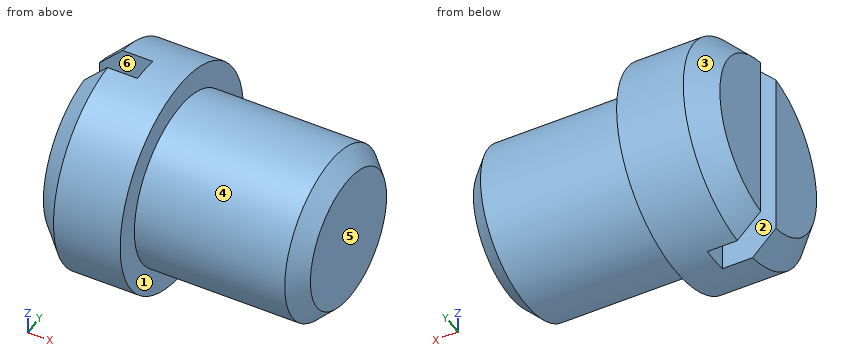
Autodesk Inventor part; units mm, degrees
ref_plane "Work Plane1" through (2.5, 0, 0) normal (0, 0, -1) x (1, 0, 0)
ref_plane "YZ Plane" through (0, 0, 0) normal (1, 0, 0) x (0, 1, 0)
ref_plane "XZ Plane" through (0, 0, 0) normal (0, 1, 0) x (-1, 0, 0)
sketch "Sketch1" plane through (0, 0, 0) normal (0, 0, 1) x (1, 0, 0)
  line L0 (-2.7, 0) -> (5, 0)
  line L1 (5, 0) -> (5, 2.5)
  line L2 (5, 2.5) -> (0, 2.5)
  line L3 (0, 2.5) -> (0, 3.25)
  line L4 (0, 3.25) -> (-2.7, 3.25)
  line L5 (-2.7, 3.25) -> (-2.7, 0)
  line L6 (-4.24, 0) -> (6.54, 0)
  line L7 (0, -0.65) -> (0, 3.9)
  dimension "d0" = 5
  dimension "d1" = 2.7
  dimension "d2" = 5
  dimension "d3" = 6.5
revolve "Body" add sketch "Sketch1" angle 360 about axis through (-2.7, 0, 0) along (1, 0, 0)
sketch "Sketch2" plane through (-2.7, 0, 0) normal (-1, 0, 0) x (0, 0, 1)
  circle A0 centre (0, 0) radius 3.25
  line L0 (-4.55, 0) -> (4.55, 0)
  line L1 (0, -4.55) -> (0, 4.55)
  line L2 (-3.25, 0.4) -> (3.25, 0.4)
  line L3 (3.25, 0.4) -> (3.25, -0.4)
  line L4 (3.25, -0.4) -> (-3.25, -0.4)
  line L5 (-3.25, -0.4) -> (-3.25, 0.4)
  line L6 (-3.25, 0) -> (3.25, 0) construction
  line L7 (0, 0.4) -> (0, -0.4) construction
  dimension "d5" = 0.8
extrude "Slot" cut sketch "Sketch2" against normal blind 1.6 contours L0 L1 L2 A0 | L3 L4 A0 | A0 L4 L1 L0 | A0 L2 L3 | L1 L4 A0 L0 | L0 A0 L2 L1 | L5 L2 A0 | A0 L4 L5
chamfer "Chamfer1" distance 0.7 angle 45 3 edges at (-2.7, -3.25, 0) (-2.7, 2.4354, -2.152) (-2.7, 2.4354, 2.152) measured on face at (-0.9, -1.3953, 2.9352)
thread "Thread"
chamfer "Chamfer2" distance 0.4908 distance2 0.4908 1 edges at (5, -2.5, 0) measured on face at (5, 0.9945, 0.5526)
ref_plane "Work Plane1" through (2.5, 0, 0) normal (0, 0, -1) x (1, 0, 0)
equation "\"d0\" = NLG"
equation "\"d1\" = KOH"
equation "\"d2\" = NND"
equation "\"d3\" = KOD"
equation "\"d5\" = SBR"
equation "\"d6\" = STI"
equation "\"d8\" = PHH"
equation "\"d16\" = PHH"
equation "\"d10\" = GEL"
equation "\"d12\" = -0.5 * GD1 + 0.5 * NND"
equation "\"d13\" = GUL"
equation "\"NND\" = 5"
equation "\"NLG\" = 5"
equation "\"GEL\" = 3.4"
equation "\"KOD\" = 6.5"
equation "\"KOH\" = 2.7"
equation "\"STI\" = 1.6"
equation "\"SBR\" = 0.8"
equation "\"GUL\" = 0.61345 * PTC"
equation "\"PHH\" = 0.7"
equation "\"GD1\" = THREADDIA - 1.2269 * PTC"
equation "\"THREADDIA\" = 5"
equation "\"TOA\" = 30deg"
equation "\"PTC\" = 0.8"
equation "\"GAL\" = 0.61345 * PTC"
properties part number "DIN 920 - M5 x 5" material "Steel, Mild"
Could you check a few things on this model? Use its own coordinates, in mm. Face numbers are marked on the shaded views. A direction names the side the tool comes from. Coordinates: 2 decimals unless noted, no trailing zeros. Order: outer loops, then holes, each group sorted by start corner. A loop starts at its lowest first (then second) coordinate and runs counter-clockwise, first axis right, second up. Notation, with made-up numbers: M 82.25,22.5 L 98.25,22.5 A16 cw 98.25,35.5 Z; hole C 45,-12.5 d6. An arc over 180 degrees is marked long. Use one line per item in the form item = value. Start each with the question number.
1. Suppose I cut it at A-A on z = 0. Write out the boundary of the cut face in (x, y), then the cut area to 3 significant figures.
2. For pin 1 (1.3 mm diameter, centred on x = -1.5, z = -0.5, fed in from +Y); pin 2 (1 mm diameter, centred on x = -1, y = 2, fed in from -Z); pin 3 (3 mm diameter, centred on x = -1, z = -2.5, fed in from -Y); pin 4 (2 mm diameter, centred on x = 1.5, y = -0.5, fed in from +Z), each with a flat end and sliding along its axis, tell me the tip position at first contact or that it passes through.
3. We'd pull the mould along Y, two halves only. Please class the marked faces 1, 2 and 3: +Y half, -Y half, draft (parallel to the pull), parting line (faces both ways), or undercut.
4. Suppose I cut it at D-D on x = 2.5. Write out the boundary of the cut face in (y, z), then the cut area to 3 significant figures.
5. On a 3-axis mill with a long thin cutter (end or side, diameter ignored), from which of +Z, -Z, +X, -X, +Y, -Y can I reach the whole of each face in a straight line? I mean the marked faces 4, 5 and 6. Say none if no direction works.
6. Please list where these lines run through material, in increasing order: line 1 (Z direction, x = 2.5, y = 0); line 2 (X direction, y = -0.25, z = -0.25); line 3 (Y direction, x = 1, z = 1.25).
7. Suppose I cut it at B-B on y = 0. Write out the boundary of the cut face in (x, z).
8. Suppose I cut it at C-C on x = -0.5. Write out the boundary of the cut face in (y, z), then the cut area to 3 significant figures.
Geometry says:
q1.outline = M -2.7,-2.55 L -2,-3.25 L 0,-3.25 L 0,-2.5 L 4.51,-2.5 L 5,-2.01 L 5,2.01 L 4.51,2.5 L 0,2.5 L 0,3.25 L -2,3.25 L -2.7,2.55 L -2.7,0.4 L -1.1,0.4 L -1.1,-0.4 L -2.7,-0.4 Z
q1.area = 40.5 mm^2
q2.pin_1 = 3.25
q2.pin_2 = -2.88
q2.pin_3 = -3.09
q2.pin_4 = 2.5
q3.face_1 = draft
q3.face_2 = undercut
q3.face_3 = +Y half
q4.outline = C 0,0 d5
q4.area = 19.6 mm^2
q5.face_4 = +X
q5.face_5 = +Z, -Z, +X, +Y, -Y
q5.face_6 = +Z, -Z, -X
q6.line_1 = -2.5 to 2.5
q6.line_2 = -1.1 to 5
q6.line_3 = -2.17 to 2.17
q7.outline = M -1.1,-3.25 L 0,-3.25 L 0,-2.5 L 4.51,-2.5 L 5,-2.01 L 5,2.01 L 4.51,2.5 L 0,2.5 L 0,3.25 L -1.1,3.25 Z
q8.outline = C 0,0 d6.5
q8.area = 33.2 mm^2
